Study the drawing (mm; zero at the part's minimum x, y, z) and answer. Coordinates: 2 decimals unless noted, no trailing zeros. Loops run counter-clockwise (first coordinate to the right, second up) from the corner with the lowest first, then second, coordinate; pieces in that order, holes last. Notation, with made-up numbers: (50, 62.5) - (78, 62.5) arc R13 ccw to (78, 72.5) - close; hole circle Ø1 at (4.5, 73). An arc over 180 degrees is marked (long way). Use one line per item in the form item = value. Start each with the question number.
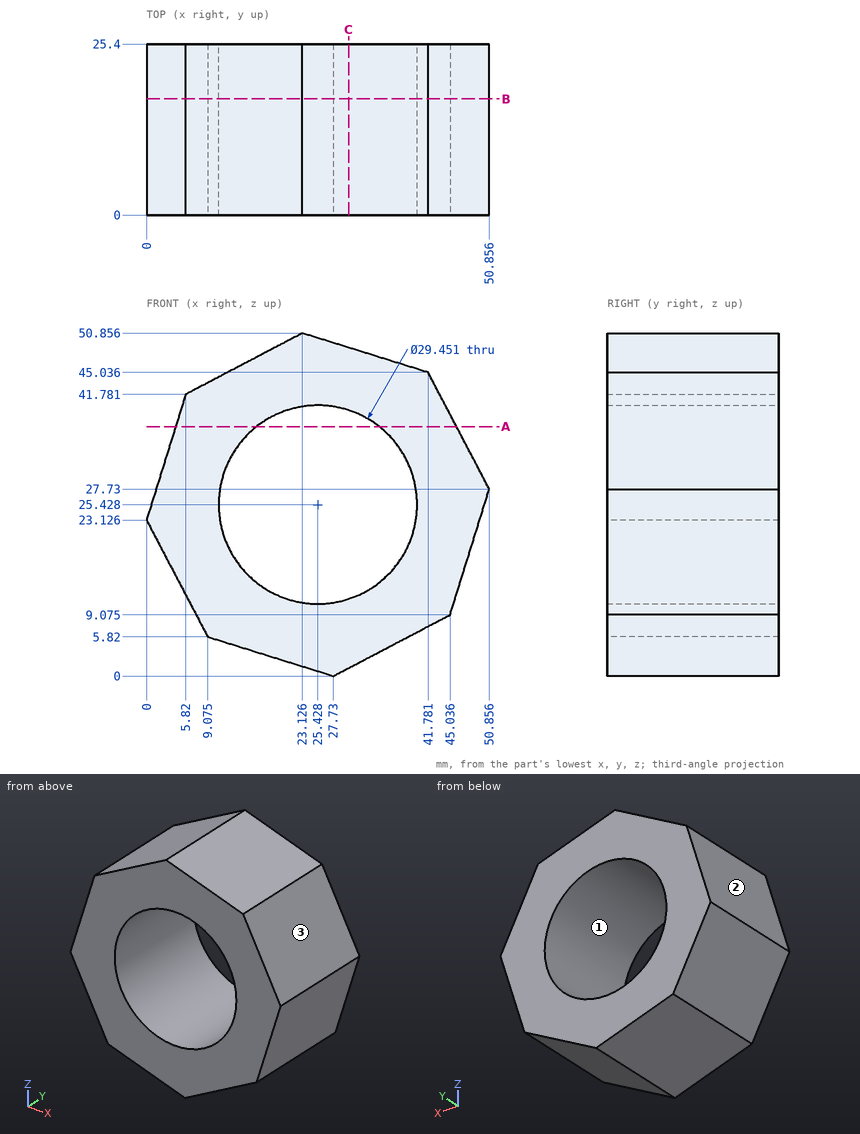
(1) Each of these flat-tipped pins is pushed along its axis until it touches: pin 1 Ø23.5 at (x, z) = (25.43, 25.43) entering from -Y; pin 2 Ø1 at (x, y) = (41, 16) entering from -Z; pin 3 Ø1 at (x, y) = (25, 5.5) entering from -Z (1 decimal); pin 4 Ø4 at (y, z) = (14.5, 39) entering from +X (1 decimal). Where does it stop, or does it pass through?
(2) Determine the mould class of the marked faces 1, 2 and 3 for opening direction X: +X half, -X half, draft (parallel to the pull), parting line (faces both ways), or undercut.
(3) A cutting plane is placed at A-A (z = 37). Determine the outline of the cut face in (x, y) (1 decimal), then the cut area to 3 significant figures.
(4) A cutting plane is placed at C-C (x = 30). Determine the outline of the cut face in (y, z).
(5) A cutting plane is placed at B-B (y = 17.25). Determine the outline of the cut face in (x, z) (1 decimal), then the cut area to 3 significant figures.
(6) Find the intervals of material crossed by probe 1 along Z at (x, y) = (34, 20.5) (1 decimal); probe 2 along Z at (x, y) = (33.5, 12) (1 decimal); probe 3 along X at (y, z) = (16.75, 18), in increasing order. Write a range as from..to.
Evaluation:
q1.pin_1 = through
q1.pin_2 = 6.7
q1.pin_3 = 0.7
q1.pin_4 = 46
q2.face_1 = undercut
q2.face_2 = -X half
q2.face_3 = +X half
q3.outline = (4.3, 0) - (16.3, 0) - (16.3, 25.4) - (4.3, 25.4) - close; (34.5, 0) - (46, 0) - (46, 25.4) - (34.5, 25.4) - close
q3.area = 596 mm^2
q4.outline = (0, 1.19) - (25.4, 1.19) - (25.4, 11.43) - (0, 11.43) - close; (0, 39.43) - (25.4, 39.43) - (25.4, 48.71) - (0, 48.71) - close
q5.outline = (0, 23.1) - (9.1, 5.8) - (27.7, 0) - (45, 9.1) - (50.9, 27.7) - (41.8, 45) - (23.1, 50.9) - (5.8, 41.8) - close; hole circle Ø29.5 at (25.4, 25.4)
q5.area = 1,160 mm^2
q6.probe_1 = 3.3..13.5, 37.4..47.5
q6.probe_2 = 3..13.1, 37.7..47.6
q6.probe_3 = 2.69..12.71, 38.14..47.82
